Could you check a few things on this model? Use its own coordinates, in mm. Coordinates: 2 decimals unless noted, no trailing zeros. Loops run counter-clockwise (first coordinate to the right, second up) from the corner with the lowest first, then second, coordinate; pieces in that order, holes last. Notation, with made-up numbers: (65, 35) - (97, 35) arc R21 cw to (97, 65) - close; hole circle Ø6 at (41, -15.5). An arc over 180 degrees is marked (long way). One line per question, with ' | ' between items. Start each with the question number.
1. I want a section at D-D, the plane y = 18.75. Write out the boundary of the cut face in (x, z) (3 decimals).
2. Please list where these lines run through material, in increasing order: L1, parallel to Y at x = 97, z = 1.75; L2, parallel to X at y = 27.75, z = 1.9; L3, parallel to X at y = 2.75, z = 2.75. Write a range as [from, to].
3. I'm going to push a flat-ended pin straight in: P1, Ø2.5, axis at x = 37.17, y = 13, coming from the -Z side. Where does the tip first touch, or does it pass through?
4. I want a section at A-A, the plane y = 3. Write out the boundary of the cut face in (x, z) (3 decimals).
5. We'd pull the mould along Y, two halves only. Please class faces 1 (the flat face through (100, 15, 2)), 2 (the flat face through (49, 0, 2)), 3 (the cylindrical face through (90.356, 13.176, 1.61)), 4 (the cylindrical face through (48.01, 15.31, 1.57)): pulls with the +Y half, pulls with the -Y half, needs draft (parallel to the pull), parting line crosses it, or undercut.
6. I want a section at C-C, the plane x = 97. Write out the boundary of the cut face in (y, z) (3 decimals), then the cut area to 3 significant figures.
7. I want a section at B-B, the plane x = 52. Write out the boundary of the cut face in (y, z) (3 decimals), then the cut area to 3 significant figures.
from build123d import *

# Parameters (mm, degrees)
SKETCH1_W             = 100
SKETCH1_H             = 30
SKETCH1_R             = 6.9977
SKETCH1_R_2           = 1.4986
SKETCH1_R_3           = 0.9906
BOSS_EXTRUDE2_DEPTH   = 3.175
F_2_56_TAPPED_HOLE1_D = 1.778
SKETCH4_R             = 4.7625
CUT_EXTRUDE1_DEPTH    = 105.45133137


with BuildPart() as part:
    # Sketch1 → Boss-Extrude2 (new body)
    with BuildSketch(Plane.XY):
        with Locations((50, 15)):
            Rectangle(SKETCH1_W, SKETCH1_H)
        with Locations((55, 15)):
            Circle(SKETCH1_R, mode=Mode.SUBTRACT)
        with Locations((37.166699296, 13)):
            Circle(SKETCH1_R_2, mode=Mode.SUBTRACT)
        with Locations((25.169778966, 20.933400182)):
            Circle(SKETCH1_R_3, mode=Mode.SUBTRACT)
    extrude(amount=BOSS_EXTRUDE2_DEPTH)

    # #2-56 Tapped Hole1 (through all)
    with Locations(Plane.XY.offset(3.175)):
        with Locations((97, 27), (97, 3), (3, 27), (3, 3), (34, 27), (34, 3)):
            Hole(F_2_56_TAPPED_HOLE1_D / 2)

    # Sketch4 → Cut-Extrude1 (cut, through all)
    with BuildSketch(Plane.XY.offset(3.175)):
        with Locations((85.9562, 15)):
            Circle(SKETCH4_R)
    extrude(amount=-CUT_EXTRUDE1_DEPTH, mode=Mode.SUBTRACT)


solid = part.part
Results are:
1) outline: (0, 0) - (49.092, 0) - (49.092, 3.175) - (0, 3.175) - close; (60.908, 0) - (83.02, 0) - (83.02, 3.175) - (60.908, 3.175) - close; (88.892, 0) - (100, 0) - (100, 3.175) - (88.892, 3.175) - close
2) L1: y = [0, 2.11], [3.89, 26.11], [27.89, 30] | L2: x = [0, 2.52], [3.48, 33.52], [34.48, 96.52], [97.48, 100] | L3: x = [0, 2.15], [3.85, 33.15], [34.85, 96.15], [97.85, 100]
3) P1: passes through
4) outline: (0, 0) - (2.111, 0) - (2.111, 3.175) - (0, 3.175) - close; (3.889, 0) - (33.111, 0) - (33.111, 3.175) - (3.889, 3.175) - close; (34.889, 0) - (96.111, 0) - (96.111, 3.175) - (34.889, 3.175) - close; (97.889, 0) - (100, 0) - (100, 3.175) - (97.889, 3.175) - close
5) face 1: needs draft | face 2: pulls with the -Y half | face 3: undercut | face 4: undercut
6) outline: (0, 0) - (2.111, 0) - (2.111, 3.175) - (0, 3.175) - close; (3.889, 0) - (26.111, 0) - (26.111, 3.175) - (3.889, 3.175) - close; (27.889, 0) - (30, 0) - (30, 3.175) - (27.889, 3.175) - close | area: 84.0 mm2
7) outline: (0, 0) - (8.678, 0) - (8.678, 3.175) - (0, 3.175) - close; (21.322, 0) - (30, 0) - (30, 3.175) - (21.322, 3.175) - close | area: 55.1 mm2
